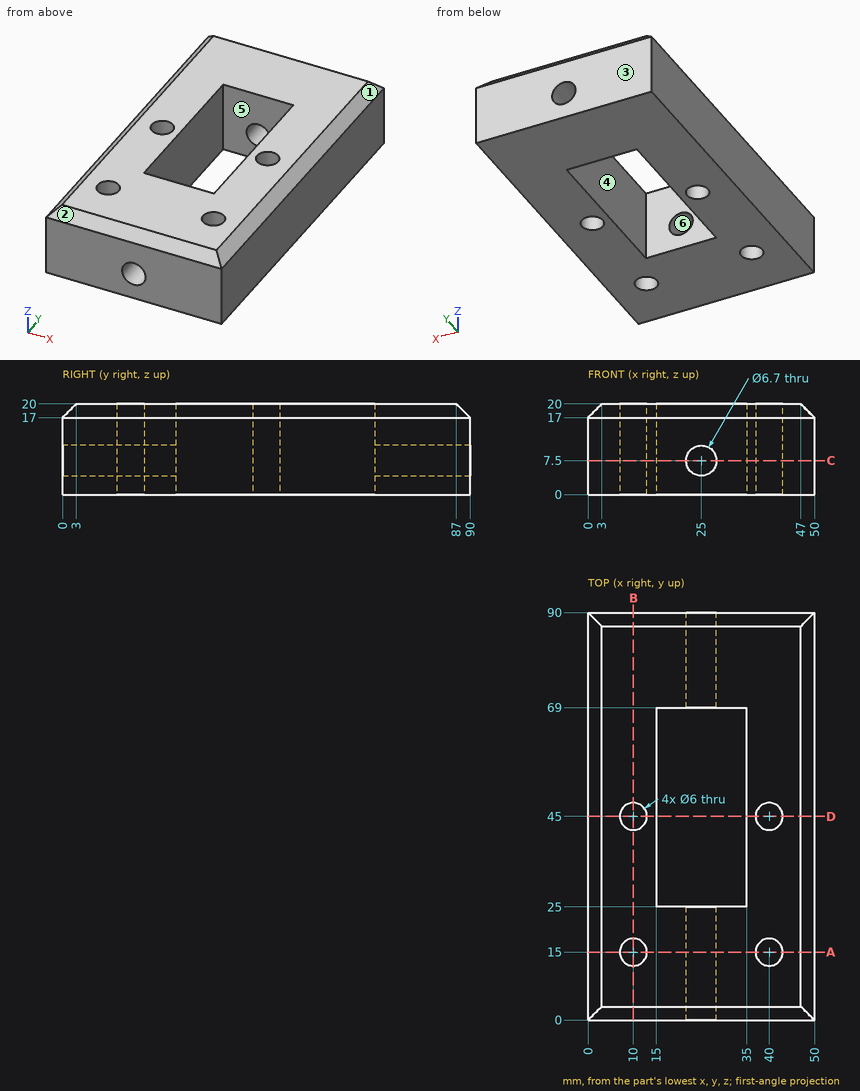
Could you check a few things on this drawing? It's one solid part, dimensions in mm from its lowest x, y, z. A direction names the side the tool comes from. Coordinates: 2 decimals unless noted, no trailing zeros. Write each loop counter-clockwise with the first axis right and the second up, starting at its lowest first coordinate (ties: lowest second). Pieces come first, ordered by that corner, then holes. Notation, with made-up numbers: (-4, 74) - (42, 74) arc R4 ccw to (42, 78) - close; hole circle Ø1 at (41.25, 80.25). An arc over 180 degrees is marked (long way). Return JSON: item names as keys, results as strings. Group by question number.
Item 1: We'd pull the mould along Y, two halves only. Please class the marked faces 1, 2, 3 and 4: pulls with the +Y half, pulls with the -Y half, needs draft (parallel to the pull), parting line crosses it, or undercut.
Item 2: Which directions (+Z, -Z, +X, -X, +Y, -Y) give clear straight access to the entire face, cutting with the end or side of a thin tool? Please do the marked faces 5 and 6.
Item 3: I'm going to push a flat-ended pin straight in: pin 1 Ø4 at (x, z) = (25, 7.5) entering from -Y. Where does the tip first touch, or does it pass through?
Item 4: If we section it at D-D (y = 45): Write out the boundary of the cut face in (x, z).
Item 5: Please list where these lines run through material, in increasing order: probe 1 along Y at (x, z) = (10, 4.75); probe 2 along X at (y, z) = (40.5, 1.75); probe 3 along Y at (x, z) = (17, 14).
Item 6: If we section it at B-B (x = 10): Write out the boundary of the cut face in (y, z), then the cut area to 3 significant figures.
Item 7: If we section it at A-A (y = 15): Write out the boundary of the cut face in (x, z), then the cut area to 3 significant figures.
Item 8: If we section it at C-C (z = 7.5): Write out the boundary of the cut face in (x, y).
Return value:
{
 "1": {"face 1": "needs draft", "face 2": "pulls with the -Y half", "face 3": "pulls with the +Y half", "face 4": "undercut"},
 "2": {"face 5": "+Z, -Z", "face 6": "+Y, -Y"},
 "3": {"pin 1": "passes through"},
 "4": {"outline": "(0, 0) - (7, 0) - (7, 20) - (3, 20) - (0, 17) - close; (13, 0) - (15, 0) - (15, 20) - (13, 20) - close; (35, 0) - (37, 0) - (37, 20) - (35, 20) - close; (43, 0) - (50, 0) - (50, 17) - (47, 20) - (43, 20) - close"},
 "5": {"probe 1": "y = 0 to 12, 18 to 42, 48 to 90", "probe 2": "x = 0 to 15, 35 to 50", "probe 3": "y = 0 to 25, 69 to 90"},
 "6": {"outline": "(0, 0) - (12, 0) - (12, 20) - (3, 20) - (0, 17) - close; (18, 0) - (42, 0) - (42, 20) - (18, 20) - close; (48, 0) - (90, 0) - (90, 17) - (87, 20) - (48, 20) - close", "area": "1,550 mm^2"},
 "7": {"outline": "(0, 0) - (7, 0) - (7, 20) - (3, 20) - (0, 17) - close; (13, 0) - (37, 0) - (37, 20) - (13, 20) - close; (43, 0) - (50, 0) - (50, 17) - (47, 20) - (43, 20) - close; hole circle Ø6.7 at (25, 7.5)", "area": "716 mm^2"},
 "8": {"outline": "(0, 0) - (21.65, 0) - (21.65, 25) - (15, 25) - (15, 69) - (21.65, 69) - (21.65, 90) - (0, 90) - close; (28.35, 0) - (50, 0) - (50, 90) - (28.35, 90) - (28.35, 69) - (35, 69) - (35, 25) - (28.35, 25) - close; hole circle Ø6 at (10, 15); hole circle Ø6 at (10, 45); hole circle Ø6 at (40, 15); hole circle Ø6 at (40, 45)"}
}
